Read the model definition and answer for the solid it produces. Units are mm, in the model's axes. Face numbers are marked on the shaded views. A direction names the side the tool comes from. Give positions to 0.01 mm unless a question says otherwise; leave off trailing zeros. Order: outer loops, then holes, each group sorted by start corner. A loop starts at its lowest first (then second) coordinate and runs counter-clockwise, first axis right, second up.
Item 1: Given pin 1 Ø2 at (x, y) = (-17.5, 8.5) entering from +Z; pin 2 Ø3 at (x, y) = (-22.5, 17) entering from -Z; pin 3 Ø12 at (x, z) = (-4.5, -9) entering from +Y, each flat-ended and moving along its own axis, determine where each tip first touches the part or whether it passes through.
Item 2: Which of the six approach directions +Z, -Z, +X, -X, +Y, -Y give full straight-line access (tool end or side, diameter ignored) to the marked faces 4, 5 and 6?
Item 3: The mould has two halves that part along X. Classify the marked faces 1, 2 and 3: +X half, -X half, draft (parallel to the pull), parting line (faces both ways), or undercut.
Item 4: A cutting plane is placed at A-A (z = -41.5). Write down the section's boundary in (x, y), plus the area to 3 significant figures.
Item 5: A cutting plane is placed at D-D (y = 2.5). Write down the section's boundary in (x, z), plus the area to 3 significant figures.
Item 6: Find the intervals of material crossed by line 1 along Z through (x, y) = (-20, 2.95); line 2 along Z through (x, y) = (-34, 11.5); line 3 along Y through (x, z) = (-8, -31), in increasing order.
Item 7: A cutting plane is placed at B-B (x = -20). Write down the section's boundary in (y, z).
Item 8: A cutting plane is placed at C-C (x = -15). Write down the section's boundary in (y, z).
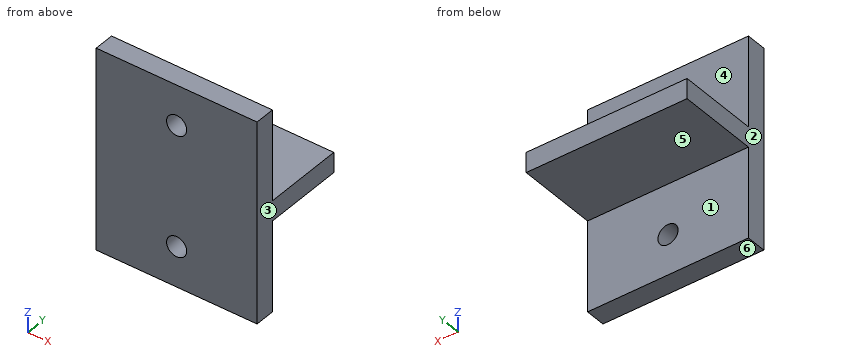
Autodesk Inventor part; units mm, degrees
ref_plane "YZ Plane" through (0, 0, 0) normal (1, 0, 0) x (0, 1, 0)
ref_plane "XZ Plane" through (0, 0, 0) normal (0, 1, 0) x (-1, 0, 0)
ref_plane "XY Plane" through (0, 0, 0) normal (0, 0, 1) x (1, 0, 0)
sketch "Sketch1" plane through (0, 0, 0) normal (0, 1, 0) x (-1, 0, 0)
  line L0 (0, 0) -> (40, 0)
  line L1 (40, 0) -> (40, -50)
  line L2 (40, -50) -> (0, -50)
  line L3 (0, -50) -> (0, 0)
  circle A0 centre (20, -10) radius 2.5
  circle A1 centre (20, -40) radius 2.5
  dimension "d0" = 40
  dimension "d1" = 50
  dimension "d2" = 5
  dimension "d3" = 5
  dimension "d4" = 10
  dimension "d5" = 10
  dimension "d6" = 20
extrude "Extrusion1" add sketch "Sketch1" along normal blind 5
sketch "Sketch2" plane through (0, 5, 0) normal (0, 1, 0) x (1, 0, 0)
  line L0 (-40, 50) -> (-40, 0)
  line L1 (0, 0) -> (0, 50)
  line L2 (-40, 22.5) -> (0, 22.5)
  line L3 (0, 22.5) -> (0, 27.5)
  line L4 (0, 27.5) -> (-40, 27.5)
  line L5 (-40, 27.5) -> (-40, 22.5)
  line L6 (-40, 0) -> (0, 0)
  point P0 (0, 22.5)
  dimension "d9" = 5
  dimension "d10" = 22.5
extrude "Extrusion2" add sketch "Sketch2" along normal blind 20 contours L4 L1 L2 L0
properties part number "LightSensor01"
Response values:
1. pin 1: stops at z = -22.5
1. pin 2: stops at z = -27.5
1. pin 3: stops at y = 5
2. face 4: +Z, +X, -X, +Y
2. face 5: -Z, +X, -X, +Y
2. face 6: -Z, +X, -X, +Y, -Y
3. face 1: draft
3. face 2: -X half
3. face 3: +X half
4. outline: (-40, 0) - (-22, 0) - (-22, 5) - (-40, 5) - close; (-18, 0) - (0, 0) - (0, 5) - (-18, 5) - close
4. area: 180 mm2
5. outline: (-40, -50) - (0, -50) - (0, 0) - (-40, 0) - close; hole circle Ø5 at (-20, -40); hole circle Ø5 at (-20, -10)
5. area: 1,960 mm2
6. line 1: z = -50 to -42.5, -37.5 to -12.5, -7.5 to 0
6. line 2: z = -27.5 to -22.5
6. line 3: y = 0 to 5
7. outline: (0, -50) - (5, -50) - (5, -42.5) - (0, -42.5) - close; (0, -37.5) - (5, -37.5) - (5, -27.5) - (25, -27.5) - (25, -22.5) - (5, -22.5) - (5, -12.5) - (0, -12.5) - close; (0, -7.5) - (5, -7.5) - (5, 0) - (0, 0) - close
8. outline: (0, -50) - (5, -50) - (5, -27.5) - (25, -27.5) - (25, -22.5) - (5, -22.5) - (5, 0) - (0, 0) - close
